from build123d import *

# Parameters (mm, degrees)
SKETCH1_W               = 254
SKETCH1_H               = 212.725
SKETCH1_W_2             = 101.6
SKETCH1_H_2             = 3.175
SKETCH1_W_3             = 50.8
SKETCH1_H_3             = 53.975
SKETCH1_W_4             = 57.15
SKETCH1_H_4             = 25.4
BOSS_EXTRUDE1_DEPTH     = 3.175
SKETCH3_W               = 38.1
SKETCH3_H               = 212.725
CUT_EXTRUDE2_DEPTH      = 4.175
FILLET1_R               = 12.7
SKETCH2_R               = 3.175
CUT_EXTRUDE1_DEPTH      = 1
CUT_EXTRUDE1_DEPTH_BACK = 4.175
FILLET2_R               = 1.5875
FILLET3_R               = 6.35


with BuildPart() as part:
    # Sketch1 → Boss-Extrude1 (new body)
    with BuildSketch(Plane(origin=(0, 0, 0), x_dir=(1, 0, 0), z_dir=(0, 1, 0))):
        Rectangle(SKETCH1_W, SKETCH1_H)
        with Locations((0, 79.248)):
            Rectangle(SKETCH1_W_2, SKETCH1_H_2, mode=Mode.SUBTRACT)
        with Locations((0, -79.248)):
            Rectangle(SKETCH1_W_2, SKETCH1_H_2, mode=Mode.SUBTRACT)
        with Locations((19.05, -6.35)):
            Rectangle(SKETCH1_W_3, SKETCH1_H_3, mode=Mode.SUBTRACT)
        with Locations((-79.375, 25.4)):
            Rectangle(SKETCH1_W_4, SKETCH1_H_4, mode=Mode.SUBTRACT)
    extrude(amount=BOSS_EXTRUDE1_DEPTH)

    # Sketch3 → Cut-Extrude2 (cut, through all)
    with BuildSketch(Plane(origin=(0, 3.175, 0), x_dir=(1, 0, 0), z_dir=(0, 1, 0))):
        with Locations((-107.95, 0)):
            Rectangle(SKETCH3_W, SKETCH3_H)
    extrude(amount=-CUT_EXTRUDE2_DEPTH, mode=Mode.SUBTRACT)

    # Fillet1
    fillet1_edges = [part.edges().sort_by_distance(p)[0] for p in [
        (127, 1.5875, 106.3625),
        (-88.9, 1.5875, -106.3625),
        (127, 1.5875, -106.3625),
        (-88.9, 1.5875, 106.3625),
    ]]
    fillet(fillet1_edges, radius=FILLET1_R)

    # Sketch2 → Cut-Extrude1 (cut, two sides)
    with BuildSketch(Plane(origin=(0, 3.175, 0), x_dir=(1, 0, 0), z_dir=(0, 1, 0))) as cut_extrude1_sk:
        with Locations((114.3, 93.5355)):
            Circle(SKETCH2_R)
        with Locations((114.3, -93.5355)):
            Circle(SKETCH2_R)
        with Locations((-76.2, -93.5355)):
            Circle(SKETCH2_R)
        with Locations((-76.2, 93.5355)):
            Circle(SKETCH2_R)
        with Locations((19.05, -93.5355)):
            Circle(SKETCH2_R)
        with Locations((19.05, 93.5355)):
            Circle(SKETCH2_R)
    extrude(amount=CUT_EXTRUDE1_DEPTH, mode=Mode.SUBTRACT)
    extrude(cut_extrude1_sk.sketch, amount=-CUT_EXTRUDE1_DEPTH_BACK, mode=Mode.SUBTRACT)

    # Fillet2
    fillet2_edges = [part.edges().sort_by_distance(p)[0] for p in [
        (-50.8, 1.5875, -12.7),
        (-50.8, 1.5875, -38.1),
    ]]
    fillet(fillet2_edges, radius=FILLET2_R)

    # Fillet3
    fillet3_edges = [part.edges().sort_by_distance(p)[0] for p in [
        (-88.9, 1.5875, -12.7),
        (-88.9, 1.5875, -38.1),
    ]]
    fillet(fillet3_edges, radius=FILLET3_R)


solid = part.part
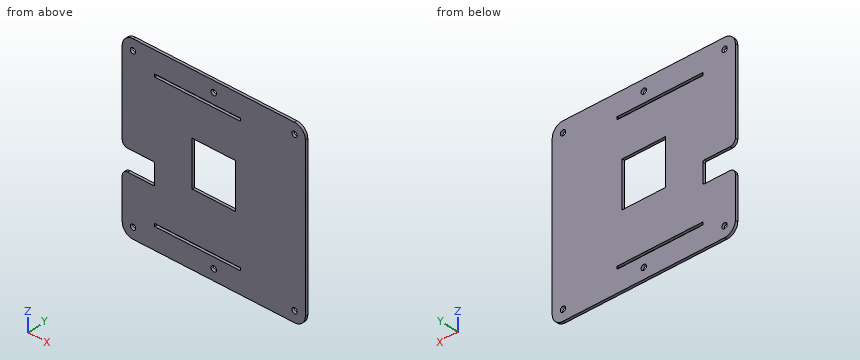
Could you check a few things on this model? Use its own coordinates, in mm. Coordinates: 2 decimals unless noted, no trailing zeros. Order: outer loops, then holes, each group sorted by start corner. A loop starts at its lowest first (then second) coordinate and runs counter-clockwise, first axis right, second up.
Q1. Please list where these lines run through material, in increasing order: L1, parallel to Z at x = -76.2, y = 2.1; L2, parallel to Z at x = 42.5, y = 0.5; L3, parallel to Z at x = 19.05, y = 2.4.
Q2. Suppose I cut it at B-B on y = 2.5. Give the number of separate pieces and of enclosed holes in the cut face, and give its area (3 significant figures).
Q3. Suppose I cut it at A-A on x = 19.05. Please give me the cut outline in (y, z) (1 decimal).
Answer:
1. L1: z = -106.36 to -96.71, -90.36 to -38.1, -12.7 to 90.36, 96.71 to 106.36
1. L2: z = -106.36 to -80.84, -77.66 to -20.64, 33.34 to 77.66, 80.84 to 106.36
1. L3: z = -106.36 to -96.71, -90.36 to -80.84, -77.66 to -20.64, 33.34 to 77.66, 80.84 to 90.36, 96.71 to 106.36
2. separate pieces: 1
2. enclosed holes: 9
2. area: 41,200 mm2
3. outline: (0, -106.4) - (3.2, -106.4) - (3.2, -96.7) - (0, -96.7) - close; (0, -90.4) - (3.2, -90.4) - (3.2, -80.8) - (0, -80.8) - close; (0, -77.7) - (3.2, -77.7) - (3.2, -20.6) - (0, -20.6) - close; (0, 33.3) - (3.2, 33.3) - (3.2, 77.7) - (0, 77.7) - close; (0, 80.8) - (3.2, 80.8) - (3.2, 90.4) - (0, 90.4) - close; (0, 96.7) - (3.2, 96.7) - (3.2, 106.4) - (0, 106.4) - close
